Could you check a few things on this drawing? It's one solid part, dimensions in mm from its lowest x, y, z. A direction names the side the tool comes from. Give positions to 0.01 mm unless a question says otherwise; leave off trailing zeros. Order: outer loops, then holes, each group sorted by start corner. A loop starts at its lowest first (then second) coordinate and runs counter-clockwise, first axis right, second up.
Item 1: I want a section at C-C, the plane z = 19. Write out the boundary of the cut face in (x, y).
Item 2: I want a section at A-A, the plane z = 14. Count the separate pieces of the cut face and the enclosed holes in it, then the cut area to 3 significant figures.
Item 3: I want a section at B-B, the plane x = 7.4. Write out the boundary of the cut face in (y, z).
Item 4: If I drill on line 1 along Y through (x, z) = (57.2, 0.6); line 2 along X through (y, z) = (18.95, 1.6); line 3 along Z through (x, y) = (86.5, 7.25), over which ranges is the centre line in solid material (lowest first)?
Item 5: I'm going to push a flat-ended pin straight in: pin 1 Ø1.5 at (x, z) = (75, 24) entering from +Y. Where does the tip first touch, or does it pass through?
Item 6: If we mould it in two halves opening along Z, with no side actions, what happens to the marked faces 1, 2 and 3? For each: +Z half, -Z half, draft (parallel to the pull), parting line (faces both ways), or undercut.
Item 7: I want a section at D-D, the plane y = 19.25. Write out the boundary of the cut face in (x, z), then the cut area to 3 significant figures.
Item 8: Which directions (+Z, -Z, +X, -X, +Y, -Y) give clear straight access to the entire face, cutting with the end or side of a thin tool? Please do the marked faces 4 and 5.
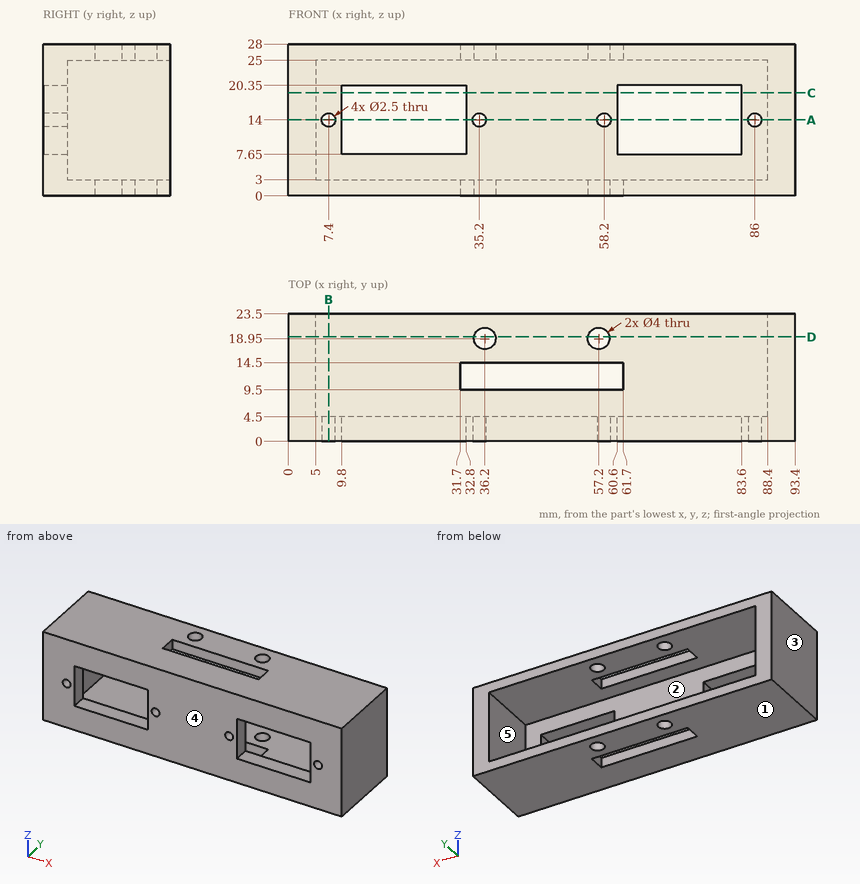
Results list:
1. outline: (0, 0) - (9.8, 0) - (9.8, 4.5) - (5, 4.5) - (5, 23.5) - (0, 23.5) - close; (32.8, 0) - (60.6, 0) - (60.6, 4.5) - (32.8, 4.5) - close; (83.6, 0) - (93.4, 0) - (93.4, 23.5) - (88.4, 23.5) - (88.4, 4.5) - (83.6, 4.5) - close
2. separate pieces: 7
2. enclosed holes: 0
2. area: 358 mm2
3. outline: (0, 0) - (23.5, 0) - (23.5, 3) - (4.5, 3) - (4.5, 12.75) - (0, 12.75) - close; (0, 15.25) - (4.5, 15.25) - (4.5, 25) - (23.5, 25) - (23.5, 28) - (0, 28) - close
4. line 1: y = 0 to 9.5, 14.5 to 16.95, 20.95 to 23.5
4. line 2: x = 0 to 34.2, 38.2 to 55.2, 59.2 to 93.4
4. line 3: z = 0 to 3, 25 to 28
5. pin 1: stops at y = 4.5
6. face 1: -Z half
6. face 2: undercut
6. face 3: draft
7. outline: (0, 0) - (34.22, 0) - (34.22, 3) - (5, 3) - (5, 25) - (34.22, 25) - (34.22, 28) - (0, 28) - close; (38.18, 0) - (55.22, 0) - (55.22, 3) - (38.18, 3) - close; (38.18, 25) - (55.22, 25) - (55.22, 28) - (38.18, 28) - close; (59.18, 0) - (93.4, 0) - (93.4, 28) - (59.18, 28) - (59.18, 25) - (88.4, 25) - (88.4, 3) - (59.18, 3) - close
7. area: 733 mm2
8. face 4: +Z, -Z, +X, -X, -Y
8. face 5: +Y
